Part model, mm, in its own coordinate system. Coordinates: 2 decimals unless noted, no trailing zeros. Loops run counter-clockwise (first coordinate to the right, second up) from the corner with the lowest first, then second, coordinate; pieces in that order, holes last. Notation, with made-up numbers: (21, -37.5) - (71, -37.5) arc R37 cw to (71, -1.5) - close; hole circle Ø4 at (-9, 73). An arc over 180 degrees is marked (long way). Use a Markdown table: item, result. Add a question column.
1) Band-saw the part on A-A (z = 0). Give the cut face in (x, y).
2) Drop flat-ended pins along their axis: P1, Ø1.5, axis at y = 2, z = -0.5, coming from the +X side; P2, Ø1, axis at y = 1.5, z = -14.5, coming from the -X side; P3, Ø10, axis at x = 16, z = 2, coming from the -Y side; P4, Ø1.5, axis at x = -12.5, y = 2, coming from the +Z side. Give the stop position or say it passes through.
3) Band-saw the part on C-C (x = -11.5). Give the cut face in (y, z).
4) Probe probe 1 along X at (y, z) = (2.35, -9); probe 2 along Z at (x, y) = (15.5, 0.5); probe 3 along Z at (x, y) = (15, 0.85). List the from-to ranges inside material, lowest first. Write a range as [from, to].
5) Band-saw the part on D-D (y = 0.8). Give the cut face in (x, z).
6) Pull direction Z, two halves, no side cores. Call faces 1 (the face through (-9.556, 1.479, 5.448)), 2 (the face through (-9, 3, 9)), 3 (the face through (6.31, 1.48, 20.03)): +Z half, -Z half, draft (parallel to the pull), parting line (faces both ways), or undercut.
7) Band-saw the part on B-B (x = 0). Give the cut face in (y, z).
from build123d import *

# Parameters (mm, degrees)
SKETCH1_R           = 21
SKETCH1_R_2         = 1.5
BOSS_EXTRUDE2_DEPTH = 3


with BuildPart() as part:
    # Sketch1 → Boss-Extrude2 (new body)
    with BuildSketch(Plane(origin=(0, 0, 0), x_dir=(1, 0, 0), z_dir=(0, 1, 0))):
        with Locations(Location((0, 0, 0), (0, 0, 270))):
            Circle(SKETCH1_R)
        with Locations(Location((-15.588457268, 9, 0), (0, 0, 270))):
            Circle(SKETCH1_R_2, mode=Mode.SUBTRACT)
        with Locations(Location((-15.588457268, -9, 0), (0, 0, 270))):
            Circle(SKETCH1_R_2, mode=Mode.SUBTRACT)
        with Locations(Location((0, -18, 0), (0, 0, 270))):
            Circle(SKETCH1_R_2, mode=Mode.SUBTRACT)
        with Locations(Location((15.588457268, -9, 0), (0, 0, 270))):
            Circle(SKETCH1_R_2, mode=Mode.SUBTRACT)
        with Locations(Location((15.588457268, 9, 0), (0, 0, 270))):
            Circle(SKETCH1_R_2, mode=Mode.SUBTRACT)
        with Locations(Location((0, 18, 0), (0, 0, 270))):
            Circle(SKETCH1_R_2, mode=Mode.SUBTRACT)
        with BuildLine():
            ThreePointArc((4.149585574, 10.187293044), (-5.5, 9.526279442), (-10.897247359, 1.5))
            Line((-10.897247359, 1.5), (-16, 1.5))
            Line((-16, 1.5), (-16, -1.5))
            Line((-16, -1.5), (-10.897247359, -1.5))
            ThreePointArc((-10.897247359, -1.5), (-9.526279442, -5.5), (-6.747661785, -8.687293044))
            Line((-6.747661785, -8.687293044), (-9.299038106, -13.106406461))
            Line((-9.299038106, -13.106406461), (-6.700961894, -14.606406461))
            Line((-6.700961894, -14.606406461), (-4.149585574, -10.187293044))
            ThreePointArc((-4.149585574, -10.187293044), (5.5, -9.526279442), (10.897247359, -1.5))
            Line((10.897247359, -1.5), (16, -1.5))
            Line((16, -1.5), (16, 1.5))
            Line((16, 1.5), (10.897247359, 1.5))
            ThreePointArc((10.897247359, 1.5), (9.526279442, 5.5), (6.747661785, 8.687293044))
            Line((6.747661785, 8.687293044), (9.299038106, 13.106406461))
            Line((9.299038106, 13.106406461), (6.700961894, 14.606406461))
            Line((6.700961894, 14.606406461), (4.149585574, 10.187293044))
        make_face(mode=Mode.SUBTRACT)
    extrude(amount=BOSS_EXTRUDE2_DEPTH)


solid = part.part
Answer block:
| question | item | result |
|---|---|---|
| 1 | outline | (-21, 0) - (-16, 0) - (-16, 3) - (-21, 3) - close; (16, 0) - (21, 0) - (21, 3) - (16, 3) - close |
| 2 | P1 | x = 21 |
| 2 | P2 | x = -15.65 |
| 2 | P3 | y = 0 |
| 2 | P4 | z = 17.41 |
| 3 | outline | (0, -17.57) - (3, -17.57) - (3, -1.5) - (0, -1.5) - close; (0, 1.5) - (3, 1.5) - (3, 17.57) - (0, 17.57) - close |
| 4 | probe 1 | [-18.97, -17.09], [-14.09, -6.32], [6.93, 14.09], [17.09, 18.97] |
| 4 | probe 2 | [-14.17, -10.5], [-7.5, -1.5], [1.5, 7.5], [10.5, 14.17] |
| 4 | probe 3 | [-14.7, -10.38], [-7.62, -1.5], [1.5, 7.62], [10.38, 14.7] |
| 5 | outline | circle Ø42 at (0, 0); hole circle Ø3 at (-15.59, -9); hole circle Ø3 at (-15.59, 9); hole (-16, -1.5) - (-10.9, -1.5) arc R11 ccw to (4.15, -10.19) - (6.7, -14.61) - (9.3, -13.11) - (6.75, -8.69) arc R11 ccw to (10.9, -1.5) - (16, -1.5) - (16, 1.5) - (10.9, 1.5) arc R11 ccw to (-4.15, 10.19) - (-6.7, 14.61) - (-9.3, 13.11) - (-6.75, 8.69) arc R11 ccw to (-10.9, 1.5) - (-16, 1.5) - close; hole circle Ø3 at (0, -18); hole circle Ø3 at (0, 18); hole circle Ø3 at (15.59, -9); hole circle Ø3 at (15.59, 9) |
| 6 | face 1 | undercut |
| 6 | face 2 | draft |
| 6 | face 3 | parting line |
| 7 | outline | (0, -21) - (3, -21) - (3, -19.5) - (0, -19.5) - close; (0, -16.5) - (3, -16.5) - (3, -11) - (0, -11) - close; (0, 11) - (3, 11) - (3, 16.5) - (0, 16.5) - close; (0, 19.5) - (3, 19.5) - (3, 21) - (0, 21) - close |
